The model under review builds one solid part; all positions refer to its coordinate system, in mm. A direction names the side the tool comes from. Give positions to 0.01 mm unless a question says otherwise; leave off trailing zeros. Write each loop counter-clockwise with the first axis right and the second up, starting at its lowest first coordinate (ties: lowest second). Pieces come first, ordered by that corner, then holes. Notation, with made-up numbers: (31.5, 84.25) - (76.5, 84.25) arc R3 cw to (76.5, 88.25) - close; hole circle Ø10 at (-12, 60.25). An arc over 180 degrees is marked (long way). Write item = value, one per line.
```python
from build123d import *

# Parameters (mm, degrees)
BOSS_EXTRUDE1_DEPTH = 70
SKETCH2_W           = 30.127897987
SKETCH2_H           = 25.625
CUT_EXTRUDE1_DEPTH  = 10
SKETCH3_W           = 36.135462637
SKETCH3_H           = 24.960917338
SKETCH3_H_2         = 26.289082662
CUT_EXTRUDE2_DEPTH  = 88.210896549
SKETCH5_W           = 40.769231001
SKETCH5_H           = 13.5
BOSS_EXTRUDE2_DEPTH = 50
SKETCH6_R           = 2
CUT_EXTRUDE3_DEPTH  = 50
FILLET1_R           = 1.25
FILLET2_R           = 16
SKETCH7_W           = 19.805527333
SKETCH7_H           = 40.769231001
CUT_EXTRUDE4_DEPTH  = 93.57213387
FILLET3_R           = 10
SKETCH9_W           = 15.47666937
SKETCH9_H           = 1.215437552
SKETCH9_W_2         = 18.289082662
SKETCH9_W_3         = 17.625
SKETCH9_H_2         = 2.622507707
SKETCH9_W_4         = 16.960917338
SKETCH9_H_3         = 1.548156683
CUT_EXTRUDE5_DEPTH  = 129.948187004
SKETCH10_W          = 7.652135561
SKETCH10_H          = 15.47666937
SKETCH10_W_2        = 8.528334289
SKETCH10_H_2        = 18.289082662
CUT_EXTRUDE8_DEPTH  = 2.75


with BuildPart() as part:
    # Sketch1 → Boss-Extrude1 (new body)
    with BuildSketch(Plane.XY):
        with BuildLine():
            Line((22.473811518, 84.75800041), (22.473811518, 83.058719541))
            ThreePointArc((22.473811518, 83.058719541), (0.883811518, 61.468719541), (22.473811518, 39.878719541))
            Line((22.473811518, 39.878719541), (22.473811518, 37.846719541))
            Line((22.473811518, 37.846719541), (-11.673355367, 37.846719541))
            Line((-11.673355367, 37.846719541), (-11.673355367, 105.594024014))
            Line((-11.673355367, 105.594024014), (1.358644633, 105.594024014))
            Line((1.358644633, 105.594024014), (1.358644633, 103.665116534))
            ThreePointArc((1.358644633, 103.665116534), (-8.83886186, 88.540693991), (9.005703845, 84.75800041))
            Line((9.005703845, 84.75800041), (22.473811518, 84.75800041))
        make_face()
    extrude(amount=-BOSS_EXTRUDE1_DEPTH)

    # Sketch2 → Cut-Extrude1 (cut)
    with BuildSketch(Plane(origin=(0, 105.594024014, 0), x_dir=(1, 0, 0), z_dir=(0, 1, 0))):
        with Locations((7.409862525, 50.9375)):
            Rectangle(SKETCH2_W, SKETCH2_H)
        with Locations((7.409862525, 19.0625)):
            Rectangle(SKETCH2_W, SKETCH2_H)
    extrude(amount=-CUT_EXTRUDE1_DEPTH, mode=Mode.SUBTRACT)

    # Sketch3 → Cut-Extrude2 (cut, through all)
    with BuildSketch(Plane(origin=(0, 84.75800041, 0), x_dir=(1, 0, 0), z_dir=(0, 1, 0))):
        with Locations((30.426375951, 51.269541331)):
            Rectangle(SKETCH3_W, SKETCH3_H)
        with Locations((30.426375951, 19.394541331)):
            Rectangle(SKETCH3_W, SKETCH3_H_2)
    extrude(amount=-CUT_EXTRUDE2_DEPTH, mode=Mode.SUBTRACT)

    # Sketch5 → Boss-Extrude2 (add)
    with BuildSketch(Plane.ZY.offset(11.673355367)):
        with Locations((20.384615501, 78.00800041)):
            Rectangle(SKETCH5_W, SKETCH5_H)
    extrude(amount=-BOSS_EXTRUDE2_DEPTH)

    # Sketch6 → Cut-Extrude3 (cut)
    with BuildSketch(Plane(origin=(0, 84.75800041, 0), x_dir=(1, 0, 0), z_dir=(0, 1, 0))):
        with Locations(Location((14.647627353, -25, 0), (0, 0, 270))):
            Circle(SKETCH6_R)
        with Locations(Location((30.329421103, -25, 0), (0, 0, 270))):
            Circle(SKETCH6_R)
    extrude(amount=-CUT_EXTRUDE3_DEPTH, mode=Mode.SUBTRACT)

    # Fillet1
    fillet1_edges = [part.edges().sort_by_distance(p)[0] for p in [
        (1.358644633, 103.665116534, -66.875),
        (22.473811518, 83.058719541, -66.875),
        (22.473811518, 39.878719541, -66.875),
        (1.358644633, 103.665116534, -35),
        (1.358644633, 103.665116534, -3.125),
        (22.473811518, 39.878719541, -35.664082662),
        (22.473811518, 39.878719541, -3.125),
        (22.473811518, 83.058719541, -35.664082662),
        (22.473811518, 83.058719541, -3.125),
    ]]
    fillet(fillet1_edges, radius=FILLET1_R)

    # Fillet2
    fillet2_edges = [part.edges().sort_by_distance(p)[0] for p in [
        (38.326644633, 78.00800041, 0),
        (38.326644633, 78.00800041, 40.769231001),
    ]]
    fillet(fillet2_edges, radius=FILLET2_R)

    # Sketch7 → Cut-Extrude4 (cut, through all)
    with BuildSketch(Plane(origin=(0, 84.75800041, 0), x_dir=(1, 0, 0), z_dir=(0, 1, 0))):
        with Locations((30.410801799, -20.384615501)):
            Rectangle(SKETCH7_W, SKETCH7_H)
    extrude(amount=-CUT_EXTRUDE4_DEPTH, mode=Mode.SUBTRACT)

    # Fillet3
    fillet3_edges = [part.edges().sort_by_distance(p)[0] for p in [
        (20.508038132, 78.00800041, 40.769231001),
    ]]
    fillet(fillet3_edges, radius=FILLET3_R)

    # Sketch9 → Cut-Extrude5 (cut, through all)
    with BuildSketch(Plane(origin=(12.358644633, 0, 0), x_dir=(0, 0, -1), z_dir=(1, 0, 0))):
        with Locations((52.096633222, 82.650281634)):
            Rectangle(SKETCH9_W, SKETCH9_H)
        with Locations((19.394541331, 82.650281634)):
            Rectangle(SKETCH9_W_2, SKETCH9_H)
        with Locations((50.9375, 102.282770161)):
            Rectangle(SKETCH9_W_3, SKETCH9_H_2)
        with Locations((19.0625, 102.282770161)):
            Rectangle(SKETCH9_W_3, SKETCH9_H_2)
        with Locations((51.269541331, 40.120797882)):
            Rectangle(SKETCH9_W_4, SKETCH9_H_3)
        with Locations((19.394541331, 40.120797882)):
            Rectangle(SKETCH9_W_2, SKETCH9_H_3)
    extrude(amount=-CUT_EXTRUDE5_DEPTH, mode=Mode.SUBTRACT)

    # Sketch10 → Cut-Extrude8 (cut)
    with BuildSketch(Plane(origin=(0, 84.75800041, 0), x_dir=(1, 0, 0), z_dir=(0, 1, 0))):
        with Locations((1.369713925, 52.096633222)):
            Rectangle(SKETCH10_W, SKETCH10_H)
        with Locations((0.931614561, 19.394541331)):
            Rectangle(SKETCH10_W_2, SKETCH10_H_2)
    extrude(amount=-CUT_EXTRUDE8_DEPTH, mode=Mode.SUBTRACT)


solid = part.part
```
1. Take a section at A-A on z = 25. Give the boundary of the cut face in (x, y).
Findings below:
outline = (-11.67, 71.26) - (12.65, 71.26) - (12.65, 84.76) - (-11.67, 84.76) - close; (16.65, 71.26) - (20.51, 71.26) - (20.51, 84.76) - (16.65, 84.76) - close
2. For line 1 (Z direction, x = 14.5, y = 84.5); line 2 (Y direction, x = 16, z = -35.5); line 3 (Y direction, x = -5, z = -27.5), list the stretches that pass through material, from the lowest coordinate up. Write a range as from..to.
Findings below:
line_1 = -70..-63.75, -38.79..-32.54, -6.25..23.01, 26.99..39.94
line_2 = 37.85..40.87, 82.07..84.76
line_3 = 37.85..39.35, 40.89..82.04, 83.26..83.69
3. Take a section at C-C on z = -34.5. Give the boundary of the cut face in (x, y).
Findings below:
outline = (-11.67, 37.85) - (22.47, 37.85) - (22.47, 38.66) arc R1.25 ccw to (21.29, 39.91) arc R21.59 cw to (21.29, 83.03) arc R1.25 ccw to (22.47, 84.27) - (22.47, 84.76) - (9.01, 84.76) arc R11 cw (long way) to (0.24, 103.61) arc R1.25 ccw to (1.36, 104.85) - (1.36, 105.59) - (-11.67, 105.59) - close
4. Take a section at B-B on y = 75. Give the boundary of the cut face in (x, z).
Findings below:
outline = (-11.67, -70) - (5.65, -70) - (5.65, 0) - (20.51, 0) - (20.51, 30.77) arc R10 ccw to (10.51, 40.77) - (-11.67, 40.77) - close; hole circle Ø4 at (14.65, 25)
5. Draft analysis for pull direction X (two halves, no side actions). For faces 5 (the flat face through (1, 84, 0)), 6 (the flat face through (20.508, 78, 16)), 7 (the flat face through (5, 84.758, 9)), state which applies: +X half, -X half, draft (parallel to the pull), parting line (faces both ways), or undercut.
Findings below:
face_5 = undercut
face_6 = +X half
face_7 = draft
6. Machinability: for faces 1 (the flat face through (-4, 104, -6.25)), 2 (the flat face through (1, 39.347, -19)), 3 (the flat face through (-1, 78, 40.769)), 4 (the flat face through (16, 39, -63.75)), which of the approach directions +Z, -Z, +X, -X, +Y, -Y give a long, thin tool a straight path to every point of the face, cutting with its end or side? Answer none if there is none.
Findings below:
face_1 = +X, +Y
face_2 = +X, -X
face_3 = +Z, +X, -X, +Y, -Y
face_4 = +X, +Y, -Y
7. Insertion check: P1, Ø7.5, axis at x = -6.5, z = -48.5, coming from the +Y side; P2, Ø5, axis at x = -3, z = -55, coming from the +Y side; P3, Ø2, axis at x = 18, y = 86, coming from the -Z side; P4, Ø16, axis at x = 6, z = 13.5, coming from the -Y side. Each pin has a flat end and moves straight along its axis. Give the tip position at first contact, or say it passes through.
Findings below:
P1 = 105.59
P2 = 84.07
P3 = through
P4 = 71.26
8. Take a section at D-D on y = 46. Give the boundary of the cut face in (x, z), and give its area (3 significant figures).
Findings below:
outline = (-11.67, -70) - (7.41, -70) - (7.41, 0) - (-11.67, 0) - close
area = 1,340 mm²
